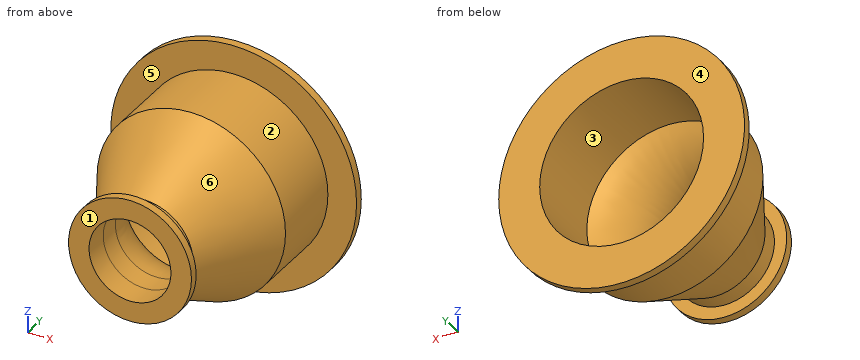
```python
from build123d import *

# Parameters (mm, degrees)
F0_R      = 29.21
F0_R_2    = 25.4
F1_DEPTH  = 25.4
F0_R_3    = 38.1
F2_DEPTH  = 2.54
F5_R      = 29.21
F4_R      = 15.24
F7_R      = 15.24
F7_R_2    = 12.7
F8_DEPTH  = 7.62
F9_R      = 19.05
F9_R_2    = 15.24
F10_DEPTH = 2.54
F11_DEPTH = 57.658


# Not quite as in the source:
# - a fillet or chamfer that OpenCascade refuses, or shapes differently, is made with other operations: its cross-section is extruded or revolved along the edge and cut away or added


with BuildPart() as f1:
    # F0 (on Front) → F1 (new body)
    with BuildSketch(Plane.XZ):
        Circle(F0_R)
        Circle(F0_R_2, mode=Mode.SUBTRACT)
    extrude(amount=F1_DEPTH)

    # F0 (on Front) → F2 (join)
    with BuildSketch(Plane.XZ):
        Circle(F0_R_3)
        Circle(F0_R, mode=Mode.SUBTRACT)
    extrude(amount=F2_DEPTH)

    # F5 (on face) → F6 section 0
    with BuildSketch(Plane.XZ.offset(25.4)):
        Circle(F5_R)
    # F4 (on offset) → F6 section 1
    with BuildSketch(Plane.XZ.offset(50.8)):
        Circle(F4_R)
    loft()

    # F7 (on face) → F8 (join)
    with BuildSketch(Plane.XZ.offset(50.8)):
        Circle(F7_R)
        Circle(F7_R_2, mode=Mode.SUBTRACT)
    extrude(amount=F8_DEPTH)

    # F9 (on face) → F10 (join)
    with BuildSketch(Plane.XZ.offset(58.42)):
        Circle(F9_R)
        Circle(F9_R_2, mode=Mode.SUBTRACT)
    extrude(amount=-F10_DEPTH)

    # F11 (cut): a face of the model
    f11_faces = [f1.faces().sort_by_distance(p)[0] for p in [
        (0, -50.8, 0),
    ]]
    extrude(f11_faces, amount=-F11_DEPTH, mode=Mode.SUBTRACT)

    # F12: fillet of radius 20.32 on 1 edges, made by hand

    # F12_s1 → F12_t2 (revolve, cut)
    with BuildSketch(Plane.XY):
        with BuildLine():
            ThreePointArc((25.4, -25.4), (16.171546065, -32.8779188315), (12.7, -44.2371441572))
            Line((12.7, -44.2371441572), (12.7, -25.4))
            Line((12.7, -25.4), (25.4, -25.4))
        make_face()
    revolve(axis=Axis((0, -25.4, 0), (0, -1, 0)), mode=Mode.SUBTRACT)


solid = f1.part
```
Check sheet for the modelled part. Datum: model origin and axes. Units: mm. Face numbers are marked on the shaded views. A direction names the side the tool comes from. Give positions to 0.01 mm unless a question says otherwise; leave off trailing zeros. Order: outer loops, then holes, each group sorted by start corner. A loop starts at its lowest first (then second) coordinate and runs counter-clockwise, first axis right, second up. Notation, with made-up numbers: (-39, 44) -> (-21, 44) arc R17 cw to (-21, 61) -> close; hole circle Ø7 at (82.25, -21). An arc over 180 degrees is marked (long way). Use CSV: the item, a comma, the result in double quotes. Start each with the question number.
1) Material ranges on line 1 (Z direction, x = 0, y = -57); line 2 (Y direction, x = 16.5, z = 28); line 3 (X direction, y = -4, z = -20), recorded low to high. Write a range as from..to.
2) Sectioned sample at C-C, the plane y = -48.5. Record the boundary of the cut face in (x, z) (3 decimals).
3) Mould release check, pull along Z, two halves, no side actions. Record for the marked faces 1, 2 and 3: released by +Z, released by -Z, zero draft, split by the parting line, or undercut.
4) Set-up check for the marked faces 4, 5 and 6: record each of +Z, -Z, +X, -X, +Y, -Y from which the full face is reachable in a straight line by a thin tool's end or side.
5) Go/stop test with flat-tipped pins: P1, Ø1, axis at x = -27.5, y = -14.5, coming from the +Z side; P2, Ø4, axis at y = -24.5, z = -11, coming from the -X side; P3, Ø8, axis at x = -13, y = -38, coming from the -Z side; P4, Ø15, axis at x = 0, z = 0, coming from the +Y side. Record where each tip stops, or that it passes through.
6) Sectioned sample at A-A, the plane x = 0. Record the boundary of the cut face in (y, z).
7) Sectioned sample at B-B, the plane y = -18.5. Record the boundary of the cut face in (x, z), plus the area to 3 significant figures.
Recorded:
1,line 1,"-19.05..-12.7, 12.7..19.05"
1,line 2,"-2.54..0"
1,line 3,"-21.29..-15.66, 15.66..21.29"
2,outline,"circle Ø33.01 at (0, 0); hole circle Ø25.4 at (0, 0)"
3,face 1,"zero draft"
3,face 2,"split by the parting line"
3,face 3,"undercut"
4,face 4,"+Z, -Z, +X, -X, +Y"
4,face 5,"-Y"
4,face 6,"none"
5,P1,"z = 11.15"
5,P2,"x = -27.79"
5,P3,"z = -21.58"
5,P4,"through"
6,outline,"(-58.42, -19.05) -> (-55.88, -19.05) -> (-55.88, -15.24) -> (-50.8, -15.24) -> (-25.4, -29.21) -> (-2.54, -29.21) -> (-2.54, -38.1) -> (0, -38.1) -> (0, -25.4) -> (-25.4, -25.4) arc R20.32 ccw to (-44.24, -12.7) -> (-58.42, -12.7) -> close; (-58.42, 12.7) -> (-44.24, 12.7) arc R20.32 ccw to (-25.4, 25.4) -> (0, 25.4) -> (0, 38.1) -> (-2.54, 38.1) -> (-2.54, 29.21) -> (-25.4, 29.21) -> (-50.8, 15.24) -> (-55.88, 15.24) -> (-55.88, 19.05) -> (-58.42, 19.05) -> close"
7,outline,"circle Ø58.42 at (0, 0); hole circle Ø50.8 at (0, 0)"
7,area,"654 mm2"
